from build123d import *

# Parameters (mm, degrees)
SKETCH2_R           = 115
BOSS_EXTRUDE3_DEPTH = 100
SKETCH3_R           = 112
CUT_EXTRUDE4_DEPTH  = 191.91883092
SKETCH4_R           = 7.5
CUT_EXTRUDE5_DEPTH  = 272.753564834
SKETCH6_W           = 24
SKETCH6_H           = 26
BOSS_EXTRUDE4_DEPTH = 2
SKETCH7_R           = 7.5
CUT_EXTRUDE6_DEPTH  = 272.753564996


with BuildPart() as part:
    # Sketch2 → Boss-Extrude3 (new body)
    with BuildSketch(Plane(origin=(0, 0, 0), x_dir=(1, 0, 0), z_dir=(0, 1, 0))):
        with Locations(Location((0, 0, 0), (0, 0, 270))):
            Circle(SKETCH2_R)
    extrude(amount=BOSS_EXTRUDE3_DEPTH)

    # Sketch3 → Cut-Extrude4 (cut, through all)
    with BuildSketch(Plane(origin=(0, 100, 0), x_dir=(1, 0, 0), z_dir=(0, 1, 0))):
        with Locations(Location((0, 0, 0), (0, 0, 270))):
            Circle(SKETCH3_R)
    extrude(amount=-CUT_EXTRUDE4_DEPTH, mode=Mode.SUBTRACT)

    # Sketch4 → Cut-Extrude5 (cut, through all)
    with BuildSketch(Plane.XY.offset(110)):
        with Locations(Location((0, 85, 0), (0, 0, 90))):
            Circle(SKETCH4_R)
    extrude(amount=CUT_EXTRUDE5_DEPTH, mode=Mode.SUBTRACT)

    # Sketch6 → Boss-Extrude4 (add)
    with BuildSketch(Plane.XY.offset(110)):
        with Locations((0.188638026, 82)):
            Rectangle(SKETCH6_W, SKETCH6_H)
    extrude(amount=BOSS_EXTRUDE4_DEPTH)

    # Sketch7 → Cut-Extrude6 (cut, through all)
    with BuildSketch(Plane(origin=(0, 0, 110), x_dir=(-1, 0, 0), z_dir=(0, 0, -1))):
        with Locations((0, 85)):
            Circle(SKETCH7_R)
    extrude(amount=-CUT_EXTRUDE6_DEPTH, mode=Mode.SUBTRACT)


solid = part.part
Could you check a few things on this model? Use its own coordinates, in mm. A direction names the side the tool comes from. Give positions to 0.01 mm unless a question says otherwise; leave off trailing zeros. Order: outer loops, then holes, each group sorted by start corner. A loop starts at its lowest first (then second) coordinate and runs counter-clockwise, first axis right, second up.
1. Suppose I cut it at C-C (x = 89.5). List the corners of the cut face in (y, z) for me, plus the area to 3 significant figures.
2. Suppose I cut it at D-D (y = 72). List the corners of the cut face in (x, z) for me.
3. Will these pins go through, and if not, where does the flat tip stop? P1, Ø10, axis at y = 29.5, z = -36, coming from the +X side; P2, Ø1, axis at y = 57, z = -28.5, coming from the -X side; P3, Ø10, axis at x = -47.5, y = 79, coming from the +Z side.
4. Suppose I cut it at A-A (x = 0). List the corners of the cut face in (y, z) for me, plus the area to 3 significant figures.
5. For faces 4 (the flat face through (-110, 100, 25)), 5 (the cylindrical face through (1.63, 77.68, 112.46)), which set-ups out of +Z, -Z, +X, -X, +Y, -Y let a thin tool reach every point of the face, with its end or its side?
6. I need wall thicknesses on L1, parallel to X at y = 35, z = 0; L2, parallel to X at y = 34, z = 3; L3, parallel to Y at x = 0, z = 113. Which ranges of each line are inside material? Lowest first, please.
7. We'd pull the mould along Z, two halves only. Please class faces 1 (the flat face through (0, 76, 110)), 2 (the cylindrical face through (-112.265, 49.3, -24.93)), 3 (the flat face through (-110, 0, 25)): pulls with the +Z half, pulls with the -Z half, needs draft (parallel to the pull), parting line crosses it, or undercut.
8. Suppose I cut it at B-B (z = -31). List the corners of the cut face in (x, y) for me, plus the area to 3 significant figures.
Solved:
1. outline: (0, -72.21) - (100, -72.21) - (100, -67.33) - (0, -67.33) - close; (0, 67.33) - (100, 67.33) - (100, 72.21) - (0, 72.21) - close
1. area: 976 mm2
2. outline: circle Ø230 at (0, 0); hole (-11.81, 110) - (-11.81, 111.38) arc R112 ccw (long way) to (12.19, 111.33) - (12.19, 110) - close
3. P1: stops at x = 110.74
3. P2: stops at x = -111.54
3. P3: stops at z = 106.86
4. outline: (0, -115) - (100, -115) - (100, -112) - (0, -112) - close; (0, 112) - (69, 112) - (69, 110) - (77.5, 110) - (77.5, 115) - (0, 115) - close; (92.5, 110) - (95, 110) - (95, 112) - (100, 112) - (100, 115) - (92.5, 115) - close
4. area: 577 mm2
5. face 4: +Z, -Z, +X, -X, +Y
5. face 5: +Z
6. L1: x = -115 to -112, 112 to 115
6. L2: x = -114.96 to -111.96, 111.96 to 114.96
6. L3: y = 0 to 77.5, 92.5 to 100
7. face 1: undercut
7. face 2: parting line crosses it
7. face 3: needs draft
8. outline: (-110.74, 0) - (-107.62, 0) - (-107.62, 100) - (-110.74, 100) - close; (107.62, 0) - (110.74, 0) - (110.74, 100) - (107.62, 100) - close
8. area: 624 mm2
